Autodesk Fusion 360 part; units mm, degrees
sketch "Sketch1" plane through (0, 0, 0) normal (0, 1, 0) x (1, 0, 0)
  line L0 (50, -50) -> (-50, -50)
  line L1 (-50, -50) -> (-50, 50)
  line L2 (-50, 50) -> (50, 50)
  line L3 (50, 50) -> (50, -50)
  line L4 (50, -50) -> (-50, 50) construction
  line L5 (-50, -50) -> (50, 50) construction
  circle A0 centre (-35, 35) radius 7.5
  circle A1 centre (-35, -35) radius 7.5
  circle A2 centre (35, -35) radius 7.5
  circle A3 centre (35, 35) radius 7.5
  circle A4 centre (0, 0) radius 25
  dimension "d1" = 100
  dimension "d2" = 100
  dimension "d3" = 15
  dimension "d4" = 15
  dimension "d5" = 50
extrude "Extrude1" add sketch "Sketch1" along normal blind 25
fillet "Fillet1" radius 15 4 edges at (-50, 12.5, 50) (-50, 12.5, -50) (50, 12.5, 50) (50, 12.5, -50)
fillet "Fillet2" radius 12.5 1 edges at (-23.3082, 25, -9.0404)
chamfer "Chamfer1" distance 5 angle 45 8 edges at (-45.6066, 25, 45.6066) (0, 25, 50) (45.6066, 25, 45.6066) (50, 25, 0) (45.6066, 25, -45.6066) (0, 25, -50) (-45.6066, 25, -45.6066) (-50, 25, 0)
delete_face "DeleteFace1" 1 faces at (36.8593, 24.9858, 1.8396)
delete_face "DeleteFace2" 8 faces at (36.0894, 22.5, -47.4524) (-11.6667, 21.6667, -48.3333) (48.3333, 21.6667, -11.6667) (47.4524, 22.5, 36.0894) (11.6667, 21.6667, 48.3333) (-36.0894, 22.5, 47.4524) (-48.3333, 21.6667, 11.6667) (-47.4524, 22.5, -36.0894)
move_face "OffsetFaces1" offset 15 1 faces at (24.8758, 16.6667, -2.4892)
For this review, take the finished solid that the model builds, in its own axes (mm). Coordinates: 2 decimals unless noted, no trailing zeros. Order: outer loops, then holes, each group sorted by start corner. A loop starts at its lowest first (then second) coordinate and runs counter-clockwise, first axis right, second up. Notation, with made-up numbers: (56.5, 77.5) -> (110.5, 77.5) arc R20 cw to (110.5, 97.5) -> close; hole circle Ø11 at (-22, -38). An arc over 180 degrees is marked (long way). Return JSON: item names as keys, results as strings.
1. For line 1 (Z direction, x = 35, y = 18.5); line 2 (Z direction, x = 32, y = 19.75); line 3 (X direction, y = 9.75, z = -4), list the stretches that pass through material, from the lowest coordinate up. Write a range as from..to.
Answer block:
{"line 1": "-50..-42.5, -27.5..27.5, 42.5..50", "line 2": "-50..-41.87, -28.13..28.13, 41.87..50", "line 3": "-50..-9.17, 9.17..50"}
2. We need section D-D on x = -33.5. Write out the cut boundary in (y, z).
Answer block:
{"outline": "(0, -50) -> (25, -50) -> (25, -42.35) -> (0, -42.35) -> close; (0, -27.65) -> (25, -27.65) -> (25, 27.65) -> (0, 27.65) -> close; (0, 42.35) -> (25, 42.35) -> (25, 50) -> (0, 50) -> close"}
3. The part is to be moulded in two halves that separate along X. For faces 1 (the cylindrical face through (-36.63, 12.32, 27.68)), 2 (the cylindrical face through (-45.72, 12.68, 45.49)), 3 (the flat face through (-1, 25, -12)), 4 (the flat face through (50, 12, 0)), say which applies: +X half, -X half, draft (parallel to the pull), parting line (faces both ways), or undercut.
Answer block:
{"face 1": "undercut", "face 2": "-X half", "face 3": "draft", "face 4": "+X half"}
4. For pin 1 Ø24 at (x, z) = (-35, 35) entering from +Y; pin 2 Ø1.5 at (y, z) = (6, 39.5) entering from +X; pin 3 Ø1.5 at (y, z) = (5.5, -37) entering from -X; pin 4 Ø13.5 at (x, z) = (-35, -35) entering from +Y, all flat-tipped, find the tip position at first contact; note any pin that passes through.
Answer block:
{"pin 1": "y = 25", "pin 2": "x = 49.52", "pin 3": "x = -49.95", "pin 4": "through"}
5. We need section C-C on y = 11. Write out the cut boundary in (x, z), and give its area (3 significant figures).
Answer block:
{"outline": "(-50, -35) arc R15 ccw to (-35, -50) -> (35, -50) arc R15 ccw to (50, -35) -> (50, 35) arc R15 ccw to (35, 50) -> (-35, 50) arc R15 ccw to (-50, 35) -> close; hole circle Ø15 at (-35, -35); hole circle Ø15 at (-35, 35); hole circle Ø20 at (0, 0); hole circle Ø15 at (35, -35); hole circle Ø15 at (35, 35)", "area": "8,790 mm²"}
6. We need section A-A on z = 0. Write out the cut boundary in (x, y).
Answer block:
{"outline": "(-50, 0) -> (-10, 0) -> (-10, 25) -> (-50, 25) -> close; (10, 0) -> (50, 0) -> (50, 25) -> (10, 25) -> close"}
7. We need section B-B on x = 0. Write out the cut boundary in (y, z).
Answer block:
{"outline": "(0, -50) -> (25, -50) -> (25, -10) -> (0, -10) -> close; (0, 10) -> (25, 10) -> (25, 50) -> (0, 50) -> close"}
